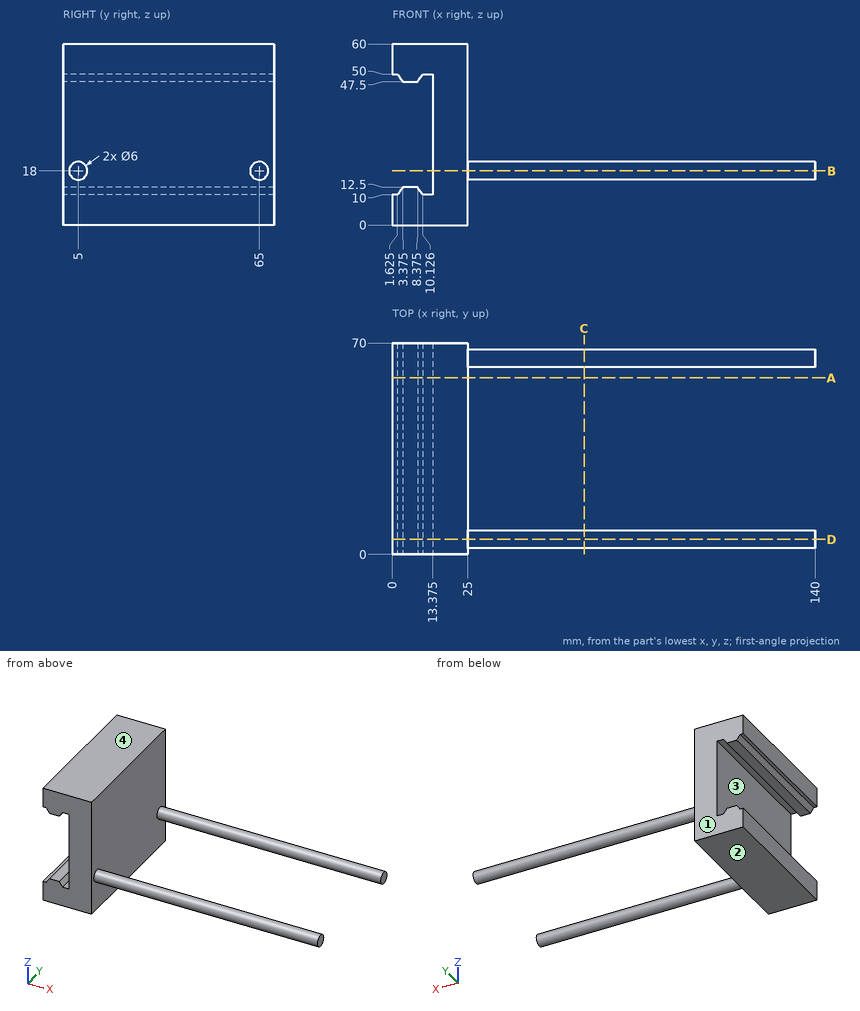
Could you check a few things on this drawing? It's one solid part, dimensions in mm from its lowest x, y, z. Coordinates: 2 decimals unless noted, no trailing zeros. Write each loop counter-clockwise with the first axis right and the second up, starting at its lowest first coordinate (ties: lowest second). Pieces come first, ordered by that corner, then holes. Notation, with made-up numbers: (-19, -11) - (29, -11) arc R12 ccw to (29, 7) - close; hole circle Ø5 at (85.5, 73). An arc over 180 degrees is marked (long way). Return JSON: item names as keys, results as strings. Group by question number.
Item 1: If we section it at D-D (y = 5): Write out the boundary of the cut face in (x, z) (1 decimal).
Item 2: If we section it at A-A (y = 58.5): Write out the boundary of the cut face in (x, z) (1 decimal).
Item 3: We'd pull the mould along Z, two halves only. Please class the marked faces 1, 2, 3 and 4: pulls with the +Z half, pulls with the -Z half, needs draft (parallel to the pull), parting line crosses it, or undercut.
Item 4: If we section it at B-B (z = 18): Write out the boundary of the cut face in (x, y) (1 decimal).
Item 5: If we section it at C-C (x = 63.5): Write out the boundary of the cut face in (y, z).
Item 6: I'm going to push flat-ended pins straight in: pin 1 Ø20 at (y, z) = (39, 21.5) entering from -X (1 decimal); pin 2 Ø5 at (y, z) = (57, 24.5) entering from +X; pin 3 Ø10 at (x, y) = (75, 59.5) entering from -Z. Where does each tip first touch, or does it pass through?
Item 7: Please list where these lines run through material, in increasing order: probe 1 along X at (y, z) = (15, 45) (1 decimal); probe 2 along X at (y, z) = (17, 52); probe 3 along Y at (x, z) = (91.5, 16) (1 decimal).
Return value:
{
 "1": {"outline": "(0, 0) - (25, 0) - (25, 15) - (140, 15) - (140, 21) - (25, 21) - (25, 60) - (0, 60) - (0, 50) - (1.6, 50) - (3.4, 47.5) - (8.4, 47.5) - (10.1, 50) - (13.4, 50) - (13.4, 10) - (10.1, 10) - (8.4, 12.5) - (3.4, 12.5) - (1.6, 10) - (0, 10) - close"},
 "2": {"outline": "(0, 0) - (25, 0) - (25, 60) - (0, 60) - (0, 50) - (1.6, 50) - (3.4, 47.5) - (8.4, 47.5) - (10.1, 50) - (13.4, 50) - (13.4, 10) - (10.1, 10) - (8.4, 12.5) - (3.4, 12.5) - (1.6, 10) - (0, 10) - close"},
 "3": {"face 1": "needs draft", "face 2": "pulls with the -Z half", "face 3": "undercut", "face 4": "pulls with the +Z half"},
 "4": {"outline": "(13.4, 0) - (25, 0) - (25, 2) - (140, 2) - (140, 8) - (25, 8) - (25, 62) - (140, 62) - (140, 68) - (25, 68) - (25, 70) - (13.4, 70) - close"},
 "5": {"outline": "circle Ø6 at (5, 18); circle Ø6 at (65, 18)"},
 "6": {"pin 1": "stops at x = 2.7", "pin 2": "stops at x = 25", "pin 3": "stops at z = 15.04"},
 "7": {"probe 1": "x = 13.4 to 25", "probe 2": "x = 0 to 25", "probe 3": "y = 2.8 to 7.2, 62.8 to 67.2"}
}
